```python
from build123d import *

# Parameters (mm, degrees)
SKETCH_1_W          = 170
SKETCH_1_H          = 38
EXTRUDE_1_DEPTH     = 4
SKETCH_2_R          = 2
CUT_EXTRUDE_1_DEPTH = 4
SKETCH_3_R          = 1.2
CUT_EXTRUDE_2_DEPTH = 10
SKETCH_4_W          = 20
SKETCH_4_H          = 17
CUT_EXTRUDE_3_DEPTH = 10
FILLET_1_R          = 2
FILLET_2_R          = 2
CUT_EXTRUDE_4_DEPTH = 10
FILLET_3_R          = 2
CUT_EXTRUDE_5_DEPTH = 10


with BuildPart() as part:
    # 草图1 → 凸台-拉伸1 (new body)
    with BuildSketch(Plane.XY):
        Rectangle(SKETCH_1_W, SKETCH_1_H)
    extrude(amount=EXTRUDE_1_DEPTH)

    # 草图2 → 切除-拉伸1 (cut)
    with BuildSketch(Plane.XY.offset(4)):
        with Locations((70, 12.5)):
            Circle(SKETCH_2_R)
        with Locations((70, -12.5)):
            Circle(SKETCH_2_R)
    cut_extrude_1 = extrude(amount=-CUT_EXTRUDE_1_DEPTH, mode=Mode.SUBTRACT)

    # 镜向1: 切除-拉伸1 across plane
    add(cut_extrude_1.mirror(Plane(origin=(0, 0, 0), x_dir=(0, 0, 1), z_dir=(1, 0, 0))), mode=Mode.SUBTRACT)

    # 草图3 → 切除-拉伸2 (cut)
    with BuildSketch(Plane.XY.offset(4)):
        with Locations((-20.295, 6.35)):
            Circle(SKETCH_3_R)
        with Locations((-20.295, -6.35)):
            Circle(SKETCH_3_R)
    extrude(amount=-CUT_EXTRUDE_2_DEPTH, mode=Mode.SUBTRACT)

    # 草图4 → 切除-拉伸3 (cut)
    with BuildSketch(Plane.XY.offset(4)):
        with Locations((-70, 0)):
            Rectangle(SKETCH_4_W, SKETCH_4_H)
    cut_extrude_3 = extrude(amount=-CUT_EXTRUDE_3_DEPTH, mode=Mode.SUBTRACT)

    # 镜向2: 切除-拉伸3 across plane
    add(cut_extrude_3.mirror(Plane(origin=(0, 0, 0), x_dir=(0, 0, 1), z_dir=(1, 0, 0))), mode=Mode.SUBTRACT)

    # 圆角1
    fillet_1_edges = [part.edges().sort_by_distance(p)[0] for p in [
        (-60, 8.5, 2),
        (-60, -8.5, 2),
        (-80, -8.5, 2),
        (-80, 8.5, 2),
        (60, -8.5, 2),
        (60, 8.5, 2),
        (80, 8.5, 2),
        (80, -8.5, 2),
    ]]
    fillet(fillet_1_edges, radius=FILLET_1_R)

    # 圆角2
    fillet_2_edges = [part.edges().sort_by_distance(p)[0] for p in [
        (85, -19, 2),
        (-85, -19, 2),
        (-85, 19, 2),
        (85, 19, 2),
    ]]
    fillet(fillet_2_edges, radius=FILLET_2_R)

    # 草图5 → 切除-拉伸4 (cut)
    with BuildSketch(Plane.XY.offset(4)):
        Polygon((-2.283893001, 13), (-17.295, -13), (12.727213998, -13), align=None)
        Polygon((4.644310229, 13), (19.655417228, -13), (34.666524227, 13), align=None)
        Polygon((41.594727457, 13), (26.583620458, -13), (56.605834456, -13), align=None)
    extrude(amount=-CUT_EXTRUDE_4_DEPTH, mode=Mode.SUBTRACT)

    # 圆角3
    fillet_3_edges = [part.edges().sort_by_distance(p)[0] for p in [
        (4.644310229, 13, 2),
        (34.666524227, 13, 2),
        (19.655417228, -13, 2),
        (41.594727457, 13, 2),
        (56.605834456, -13, 2),
        (26.583620458, -13, 2),
        (-2.283893001, 13, 2),
        (12.727213998, -13, 2),
        (-17.295, -13, 2),
    ]]
    fillet(fillet_3_edges, radius=FILLET_3_R)

    # 草图6 → 切除-拉伸5 (cut)
    with BuildSketch(Plane.XY.offset(4)):
        with BuildLine():
            Line((-55, -11.2), (-55, 11.2))
            ThreePointArc((-55, 11.2), (-52.2, 14), (-49.4, 11.2))
            Line((-49.4, 11.2), (-49.4, -11.2))
            ThreePointArc((-49.4, -11.2), (-52.2, -14), (-55, -11.2))
        make_face()
        with BuildLine():
            Line((-43.4, -11.2), (-43.4, 11.2))
            ThreePointArc((-43.4, 11.2), (-40.6, 14), (-37.8, 11.2))
            Line((-37.8, 11.2), (-37.8, -11.2))
            ThreePointArc((-37.8, -11.2), (-40.6, -14), (-43.4, -11.2))
        make_face()
        with BuildLine():
            Line((-31.8, -11.2), (-31.8, 11.2))
            ThreePointArc((-31.8, 11.2), (-29, 14), (-26.2, 11.2))
            Line((-26.2, 11.2), (-26.2, -11.2))
            ThreePointArc((-26.2, -11.2), (-29, -14), (-31.8, -11.2))
        make_face()
    extrude(amount=-CUT_EXTRUDE_5_DEPTH, mode=Mode.SUBTRACT)


solid = part.part
```
For this review, take the finished solid that the model builds, in its own axes (mm). A direction names the side the tool comes from. Round coordinates to 2 decimals unless told otherwise and drop trailing zeros. Write each loop counter-clockwise with the first axis right and the second up, starting at its lowest first coordinate (ties: lowest second). Pieces come first, ordered by that corner, then holes. Notation, with made-up numbers: (6, 14.5) - (59, 14.5) arc R30 ccw to (59, 44.5) - close; hole circle Ø8 at (50, -5.75). An arc over 180 degrees is marked (long way). Answer as CSV lines item,"result". Start each with the question number.
(1) Add section B-B, the plane x = -70. State the section outline as (y, z) points.
(2) Machinability: for faces 1 (the flat face through (-1, -19, 2)), 2 (the flat face through (70, 8.5, 2)), which of the approach directions +Z, -Z, +X, -X, +Y, -Y give a long, thin tool a straight path to every point of the face, cutting with its end or side? Answer none if there is none.
(3) Add section C-C, the plane y = -3. State how many separate pieces and enclosed holes the cut face has, plus the area to 3 significant figures.
(4) For line 1 (Y direction, x = 70, z = 2.25); line 2 (Y direction, x = -7.5, z = 1.65); line 3 (Y direction, x = 71.5, z = 1.15), list the stretches that pass through material, from the lowest coordinate up.
(5) Mouldability with a two-part tool opening along X and no side actions: class faces 3 (the flat face through (85, 0, 2)), 4 (the cylindrical face through (-29, 14, 2)), 5 (the flat face through (-1, 19, 2)) as +X half, -X half, draft (parallel to the pull), parting line (faces both ways), or undercut.
(6) Add section A-A, the plane x = -52.2. State the section outline as (y, z) points, plus the area to 3 significant figures.
(7) For pin 1 (4 mm diameter, centred on x = -56.5, y = 10, fed in from -Z); pin 2 (3.5 mm diameter, centred on x = -70, y = 12.5, fed in from -Z), all flat-tipped, find the tip position at first contact; note any pin that passes through.
From the geometry:
1,outline,"(-19, 0) - (-14.5, 0) - (-14.5, 4) - (-19, 4) - close; (-10.5, 0) - (-8.5, 0) - (-8.5, 4) - (-10.5, 4) - close; (8.5, 0) - (10.5, 0) - (10.5, 4) - (8.5, 4) - close; (14.5, 0) - (19, 0) - (19, 4) - (14.5, 4) - close"
2,face 1,"+Z, -Z, +X, -X, -Y"
2,face 2,"+Z, -Z"
3,separate pieces,"9"
3,enclosed holes,"0"
3,area,"259 mm²"
4,line 1,"y = -19 to -14.5, -10.5 to -8.5, 8.5 to 10.5, 14.5 to 19"
4,line 2,"y = -19 to -13, 3.97 to 19"
4,line 3,"y = -19 to -13.82, -11.18 to -8.5, 8.5 to 11.18, 13.82 to 19"
5,face 3,"+X half"
5,face 4,"undercut"
5,face 5,"draft"
6,outline,"(-19, 0) - (-14, 0) - (-14, 4) - (-19, 4) - close; (14, 0) - (19, 0) - (19, 4) - (14, 4) - close"
6,area,"40.0 mm²"
7,pin 1,"stops at z = 0"
7,pin 2,"passes through"
